from build123d import *

# Parameters (mm, degrees)
SKETCH1_R           = 8
SKETCH1_R_2         = 5
BOSS_EXTRUDE1_DEPTH = 7.5
CHAMFER1_SIZE       = 1
CHAMFER1_SIZE2      = 1.732050808
CHAMFER2_SIZE       = 0.5
CHAMFER3_SIZE       = 0.2
CUT_EXTRUDE1_START  = -3.230304
SKETCH2_R           = 1.5
CUT_EXTRUDE1_DEPTH  = 3.230304
CIRPATTERN1_COUNT   = 2
CIRPATTERN1_ANGLE   = 90


with BuildPart() as part:
    # Sketch1 → Boss-Extrude1 (new body)
    with BuildSketch(Plane(origin=(0, 0, 0), x_dir=(1, 0, 0), z_dir=(0, 1, 0))):
        Circle(SKETCH1_R)
        Circle(SKETCH1_R_2, mode=Mode.SUBTRACT)
    extrude(amount=BOSS_EXTRUDE1_DEPTH)

    # Chamfer1
    chamfer1_edges = [part.edges().sort_by_distance(p)[0] for p in [
        (-8, 7.5, 0),
    ]]
    chamfer1_side = [part.faces().sort_by_distance(p)[0] for p in [
        (-8, 3.75, 0),
    ]]
    chamfer(chamfer1_edges, length=CHAMFER1_SIZE, length2=CHAMFER1_SIZE2, reference=chamfer1_side[0])

    # Chamfer2
    chamfer2_edges = [part.edges().sort_by_distance(p)[0] for p in [
        (-8, 0, 0),
    ]]
    chamfer(chamfer2_edges, length=CHAMFER2_SIZE)

    # Chamfer3
    chamfer3_edges = [part.edges().sort_by_distance(p)[0] for p in [
        (-5, 0, 0),
    ]]
    chamfer(chamfer3_edges, length=CHAMFER3_SIZE)

    # Sketch2 → Cut-Extrude1 (cut)
    with BuildSketch(Plane(origin=(8, 0, 0), x_dir=(0, 0, -1), z_dir=(1, 0, 0)).offset(CUT_EXTRUDE1_START)):
        with Locations((0, 3.5)):
            Circle(SKETCH2_R)
    cut_extrude1 = extrude(amount=CUT_EXTRUDE1_DEPTH, mode=Mode.SUBTRACT)

    # CirPattern1: Cut-Extrude1 ×2 about axis
    cirpattern1_axis = Axis((0, 7.5, 0), (0, 1, 0))
    for i in range(1, CIRPATTERN1_COUNT):
        add(cut_extrude1.rotate(cirpattern1_axis, i * CIRPATTERN1_ANGLE / (CIRPATTERN1_COUNT - 1)), mode=Mode.SUBTRACT)


solid = part.part
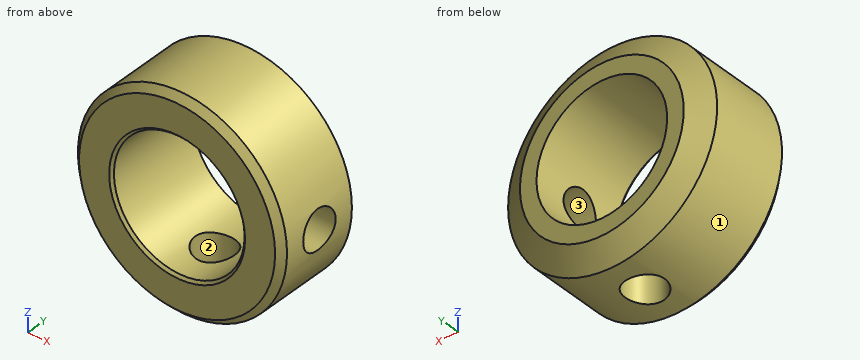
Here's how the part is built. I have some questions about the finished solid (model axes, mm). Face numbers are marked on the shaded views. Round coordinates to 2 decimals unless told otherwise and drop trailing zeros. Order: outer loops, then holes, each group sorted by start corner. A loop starts at its lowest first (then second) coordinate and runs counter-clockwise, first axis right, second up. Notation, with made-up numbers: (-8.75, 27.25) -> (23.25, 27.25) arc R16 ccw to (23.25, 35.25) -> close; hole circle Ø3 at (44.5, 10.5). An arc over 180 degrees is marked (long way). Use CSV: the item, a comma, the result in double quotes.
1. I want a section at A-A on z = 0. List the corners of the cut face in (x, y) for me.
Recorded:
outline,"(-8, 0.5) -> (-7.5, 0) -> (-5.2, 0) -> (-5, 0.2) -> (-5, 7.5) -> (-6.27, 7.5) -> (-8, 6.5) -> close; (5, 0.2) -> (5.2, 0) -> (7.5, 0) -> (8, 0.5) -> (8, 2) -> (5, 2) -> close; (5, 5) -> (8, 5) -> (8, 6.5) -> (6.27, 7.5) -> (5, 7.5) -> close"
2. I want a section at C-C on y = 1.5. List the corners of the cut face in (x, z) for me.
Recorded:
outline,"circle Ø16 at (0, 0); hole circle Ø10 at (0, 0)"
3. Thinking about a two-plate mould opening in X: for the marked faces 1, 2 and 3, which applies, pulls with the +X half, pulls with the -X half, needs draft (parallel to the pull), parting line crosses it, or undercut?
Recorded:
face 1,"parting line crosses it"
face 2,"undercut"
face 3,"needs draft"
4. I want a section at B-B on y = 4.5. List the corners of the cut face in (x, z) for me.
Recorded:
outline,"(-1.12, -7.92) -> (-1.12, -4.87) arc R5 cw (long way) to (4.87, 1.12) -> (7.92, 1.12) arc R8 ccw (long way) to start; (1.12, -7.92) arc R8 ccw to (7.92, -1.12) -> (4.87, -1.12) arc R5 cw to (1.12, -4.87) -> close"
5. I'm going to push flat-ended pins straight in: P1, Ø1, axis at x = 3.5, y = 4, coming from the +Z side; P2, Ø6, axis at x = 0, z = 0, coming from the +Y side; P3, Ø3, axis at y = 2, z = -2, coming from the +X side; P4, Ø4, axis at x = 3.5, y = 2, coming from the +Z side. Where does each tip first touch, or does it pass through?
Recorded:
P1,"stops at z = 7.42"
P2,"passes through"
P3,"stops at x = 7.98"
P4,"stops at z = 7.86"
6. I want a section at D-D on y = 3.5. List the corners of the cut face in (x, z) for me, and give its area (3 significant figures).
Recorded:
outline,"(-1.5, -7.86) -> (-1.5, -4.77) arc R5 cw (long way) to (4.77, 1.5) -> (7.86, 1.5) arc R8 ccw (long way) to start; (1.5, -7.86) arc R8 ccw to (7.86, -1.5) -> (4.77, -1.5) arc R5 cw to (1.5, -4.77) -> close"
area,"104 mm2"
7. I need wall thicknesses on line 1 along Y through (x, z) = (5.7, 0); line 2 along X through (y, z) = (3.75, 0); line 3 along X through (y, z) = (5.75, -4.5). Which ranges of each line are inside material? Lowest first, please.
Recorded:
line 1,"y = 0 to 2, 5 to 7.5"
line 2,"x = -8 to -5"
line 3,"x = -6.61 to -2.18, 2.18 to 6.61"
